For this review, take the finished solid that the model builds, in its own axes (mm). Coordinates: 2 decimals unless noted, no trailing zeros. Write each loop counter-clockwise with the first axis right and the second up, starting at its lowest first coordinate (ties: lowest second). Pieces come first, ordered by that corner, then holes. Notation, with made-up numbers: (-36, 59.25) - (-27, 59.25) arc R11 cw to (-27, 65.25) - close; hole circle Ø11 at (-27.75, -23.5). An arc over 180 degrees is marked (long way). Write each question's results on one line, items separated by ' | '.
from build123d import *

# Parameters (mm, degrees)
SKETCH1_R           = 1.5
BOSS_EXTRUDE1_DEPTH = 6.35


with BuildPart() as part:
    # Sketch1 → Boss-Extrude1 (new body)
    with BuildSketch(Plane(origin=(0, 0, 0), x_dir=(1, 0, 0), z_dir=(0, 1, 0))):
        with BuildLine():
            Line((-70, -100), (70, -100))
            ThreePointArc((70, -100), (91.213203436, -91.213203436), (100, -70))
            Line((100, -70), (100, 70))
            ThreePointArc((100, 70), (91.213203436, 91.213203436), (70, 100))
            Line((70, 100), (-70, 100))
            ThreePointArc((-70, 100), (-91.213203436, 91.213203436), (-100, 70))
            Line((-100, 70), (-100, -70))
            ThreePointArc((-100, -70), (-91.213203436, -91.213203436), (-70, -100))
        make_face()
        with Locations((75, 75)):
            Circle(SKETCH1_R, mode=Mode.SUBTRACT)
        with Locations((65, 65)):
            Circle(SKETCH1_R, mode=Mode.SUBTRACT)
        with Locations((65, -65)):
            Circle(SKETCH1_R, mode=Mode.SUBTRACT)
        with Locations((75, -75)):
            Circle(SKETCH1_R, mode=Mode.SUBTRACT)
        with Locations((-65, -65)):
            Circle(SKETCH1_R, mode=Mode.SUBTRACT)
        with Locations((-75, -75)):
            Circle(SKETCH1_R, mode=Mode.SUBTRACT)
        with Locations((-65, 65)):
            Circle(SKETCH1_R, mode=Mode.SUBTRACT)
        with Locations((-75, 75)):
            Circle(SKETCH1_R, mode=Mode.SUBTRACT)
    extrude(amount=BOSS_EXTRUDE1_DEPTH)


solid = part.part
Q1. Take a section at B-B on z = -80. State the section outline as (x, y) points.
Results found:
outline: (-98.28, 0) - (98.28, 0) - (98.28, 6.35) - (-98.28, 6.35) - close
Q2. Take a section at A-A on y = 2. State how many separate pieces and enclosed holes the cut face has, plus the area to 3 significant figures.
Results found:
separate pieces: 1 | enclosed holes: 8 | area: 39,200 mm2
Q3. Wall thickness on line 1 along Z through (x, y) = (65, 2.5); line 2 along Z through (x, y) = (75, 1.5): over which ranges is each line inside the solid? List them lowest first. Write a range as from..to.
Results found:
line 1: -100..-66.5, -63.5..63.5, 66.5..100 | line 2: -99.58..-76.5, -73.5..73.5, 76.5..99.58
